Could you check a few things on this model? Use its own coordinates, in mm. Give positions to 0.01 mm unless a question says otherwise; leave off trailing zeros. Order: outer loops, then holes, each group sorted by start corner. A loop starts at its lowest first (then second) coordinate and runs counter-clockwise, first axis right, second up. Notation, with made-up numbers: (24, 79) - (28, 79) arc R31 ccw to (28, 115) - close; hole circle Ø3 at (-24, 66.25). An arc over 180 degrees is marked (long way). Put each result on its own line as item: value.
from build123d import *

# Parameters (mm, degrees)
SKETCH_1_W      = 24.2
SKETCH_1_H      = 23.5
EXTRUDE_1_DEPTH = 3


with BuildPart() as part:
    # 草图1 → 凸台-拉伸1 (new body)
    with BuildSketch(Plane.XY):
        Polygon((-30.949264706, 17.967420182), (-15.349264706, 17.967420182), (-15.349264706, -8.713823312), (-15.349264706, -72.032579818), (34.650735294, -72.032579818), (34.650735294, -8.713823312), (34.650735294, 17.967420182), (49.050735294, 17.967420182), (49.050735294, -132.032579818), (33.550735294, -132.032579818), (33.550735294, -158.532579818), (-5.449264706, -158.532579818), (-5.449264706, -132.032579818), (-30.949264706, -132.032579818), align=None)
        with BuildLine():
            Line((-17.749264706, 12.967420182), (-17.749264706, -7.032579818))
            ThreePointArc((-17.749264706, -7.032579818), (-19.349264706, -8.632579818), (-20.949264706, -7.032579818))
            Line((-20.949264706, -7.032579818), (-20.949264706, 12.967420182))
            ThreePointArc((-20.949264706, 12.967420182), (-19.349264706, 14.567420182), (-17.749264706, 12.967420182))
        make_face(mode=Mode.SUBTRACT)
        with BuildLine():
            Line((37.050735294, 12.967420182), (37.050735294, -7.032579818))
            ThreePointArc((37.050735294, -7.032579818), (38.650735294, -8.632579818), (40.250735294, -7.032579818))
            Line((40.250735294, -7.032579818), (40.250735294, 12.967420182))
            ThreePointArc((40.250735294, 12.967420182), (38.650735294, 14.567420182), (37.050735294, 12.967420182))
        make_face(mode=Mode.SUBTRACT)
        with Locations((9.650735294, -143.782579818)):
            Rectangle(SKETCH_1_W, SKETCH_1_H, mode=Mode.SUBTRACT)
    extrude(amount=EXTRUDE_1_DEPTH)


solid = part.part
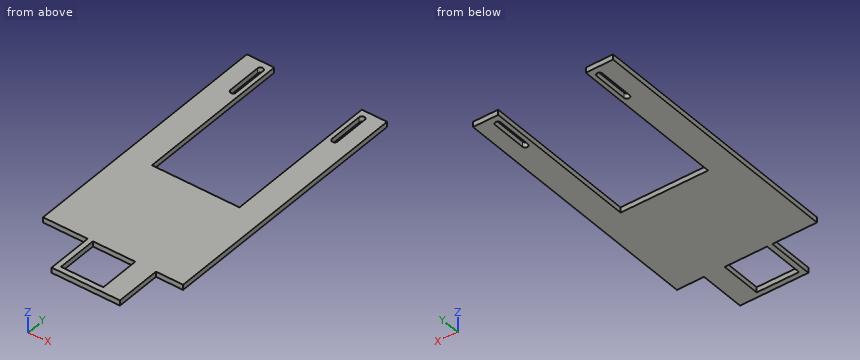
1) I'm going to push flat-ended pins straight in: pin 1 (0.9 mm diameter, centred on y = -145.5, z = 1.5, fed in from -X); pin 2 (0.9 mm diameter, centred on x = 43, z = 1.5, fed in from -Y); pin 3 (1.5 mm diameter, centred on y = -146, z = 1, fed in from +X); pin 4 (12 mm diameter, centred on x = -7, y = -31.5, fed in from -Z). Where does each tip first touch, or does it pass through?
Filled in:
pin 1: stops at x = -5.45
pin 2: stops at y = -132.03
pin 3: stops at x = 33.55
pin 4: passes through
2) If I drill on line 1 (X direction, y = 4, z = 1.7); line 2 (X direction, y = -58, z = 0.8); line 3 (Y direction, x = 20.5, z = 1.45), over which ranges is the centre line in solid material (lowest first)? Write a range as [from, to].
Filled in:
line 1: x = [-30.95, -20.95], [-17.75, -15.35], [34.65, 37.05], [40.25, 49.05]
line 2: x = [-30.95, -15.35], [34.65, 49.05]
line 3: y = [-158.53, -155.53], [-132.03, -72.03]
3) Suppose I cut it at A-A, the plane x = 12.5. List the corners of the cut face in (y, z) for me.
Filled in:
outline: (-158.53, 0) - (-155.53, 0) - (-155.53, 3) - (-158.53, 3) - close; (-132.03, 0) - (-72.03, 0) - (-72.03, 3) - (-132.03, 3) - close
4) Suppose I cut it at D-D, the plane x = 32. List the corners of the cut face in (y, z) for me, and give its area (4 significant figures).
Filled in:
outline: (-158.53, 0) - (-72.03, 0) - (-72.03, 3) - (-158.53, 3) - close
area: 259.5 mm^2
5) Suppose I cut it at C-C, the plane z = 0.65. List the corners of the cut face in (x, y) for me.
Filled in:
outline: (-30.95, -132.03) - (-5.45, -132.03) - (-5.45, -158.53) - (33.55, -158.53) - (33.55, -132.03) - (49.05, -132.03) - (49.05, 17.97) - (34.65, 17.97) - (34.65, -72.03) - (-15.35, -72.03) - (-15.35, 17.97) - (-30.95, 17.97) - close; hole (-20.95, -7.03) arc R1.6 ccw to (-17.75, -7.03) - (-17.75, 12.97) arc R1.6 ccw to (-20.95, 12.97) - close; hole (-2.45, -155.53) - (21.75, -155.53) - (21.75, -132.03) - (-2.45, -132.03) - close; hole (37.05, -7.03) arc R1.6 ccw to (40.25, -7.03) - (40.25, 12.97) arc R1.6 ccw to (37.05, 12.97) - close
6) Suppose I cut it at B-B, the plane y = -49. List the corners of the cut face in (x, z) for me, and give its area (3 significant figures).
Filled in:
outline: (-30.95, 0) - (-15.35, 0) - (-15.35, 3) - (-30.95, 3) - close; (34.65, 0) - (49.05, 0) - (49.05, 3) - (34.65, 3) - close
area: 90.0 mm^2
